Could you check a few things on this model? Use its own coordinates, in mm. A direction names the side the tool comes from. Coordinates: 2 decimals unless noted, no trailing zeros. Write each loop counter-clockwise with the first axis right and the second up, starting at its lowest first coordinate (ties: lowest second). Pieces come first, ordered by that corner, then holes. Notation, with made-up numbers: M 38,-9 L 82,-9 A20 ccw 82,18 Z; hole C 38,72 d2. An arc over 180 degrees is marked long. Answer as CSV lines item,"result". Start each with the question number.
Item 1: We'd pull the mould along X, two halves only. Please class faces 6 (the cylindrical face through (13.117, 2.07, 26.74)), 7 (the flat face through (-18.121, -3, 13)), 8 (the flat face through (-18.283, 2.3, 12.8)): +X half, -X half, draft (parallel to the pull), parting line (faces both ways), or undercut.
Item 2: On a 3-axis mill with a long thin cutter (end or side, diameter ignored), from which of +Z, -Z, +X, -X, +Y, -Y can I reach the whole of each face in a straight line? I mean faces 1 (the flat face through (-21, 1.131, 13)), 2 (the cylindrical face through (-13, -3, 3)), 3 (the flat face through (9.917, 0, 13)), 4 (the flat face through (-4, 1.907, 13)), 5 (the flat face through (-20, 2.733, 13)). Say none if no direction works.
Item 3: Suppose I cut it at C-C, the plane x = 4.5. Write out the boundary of the cut face in (y, z), and give its area (3 significant figures).
Item 4: Suppose I cut it at B-B, the plane y = -4. Write out the boundary of the cut face in (x, z).
Item 5: If I drill on line 1 along Z through (x, y) = (-7, 1.5); line 2 along Y through (x, z) = (-15.5, 23.75); line 3 along X through (y, z) = (0, 18.25), over which ranges is the centre line in solid material (lowest first)? Write a range as [from, to].
Item 6: Suppose I cut it at D-D, the plane x = -11. Write out the boundary of the cut face in (y, z), and give its area (3 significant figures).
Item 7: I'm going to push flat-ended pins straight in: P1, Ø3.5, axis at x = -12.5, y = 0.5, coming from the -Z side; P2, Ø3, axis at x = 8.5, z = 16, coming from the -Y side; P3, Ø2.5, axis at x = -22, z = 8.5, coming from the -Y side. Where does each tip first touch, or does it pass through?
Item 8: Suppose I cut it at A-A, the plane x = -17. Write out the boundary of the cut face in (y, z).
```python
from build123d import *

# Parameters (mm, degrees)
BOSS_EXTRUDE3_DEPTH = 26
FILLET6_START       = -1
FILLET6_DEPTH       = 28
BOSS_EXTRUDE5_DEPTH = 4
SKETCH6_R           = 0.5
BOSS_EXTRUDE6_DEPTH = 1.5
LPATTERN1_COUNT     = 2
LPATTERN1_PITCH     = 27.5


with BuildPart() as part:
    # Sketch4 → Boss-Extrude3 (new body)
    with BuildSketch(Plane.XY):
        with BuildLine():
            Line((-18.782676832, -0.738323828), (9.917323168, -0.738323828))
            Line((9.917323168, -0.738323828), (9.917323168, 0.761676172))
            Line((9.917323168, 0.761676172), (14.217323168, 0.761676172))
            Line((14.217323168, 0.761676172), (14.217323168, 3.761676172))
            Line((14.217323168, 3.761676172), (10.417323168, 3.761676172))
            Line((10.417323168, 3.761676172), (10.417323168, 1.907320096))
            Line((10.417323168, 1.907320096), (-18.282676832, 1.907320096))
            Line((-18.282676832, 1.907320096), (-18.282676832, 2.732812963))
            Line((-18.282676832, 2.732812963), (-21.829938074, 2.732812963))
            ThreePointArc((-21.829938074, 2.732812963), (-22.961793852, 2.121559656), (-23.782676832, 1.131166179))
            Line((-23.782676832, 1.131166179), (-18.782676832, 1.131166179))
            Line((-18.782676832, 1.131166179), (-18.782676832, -0.738323828))
        make_face()
    extrude(amount=BOSS_EXTRUDE3_DEPTH)

    # Fillet6: read off the stored shape, not the designer's step
    # Fillet6 outline → Fillet6 (cut)
    with BuildSketch(Plane.XY.offset(FILLET6_START)):
        with BuildLine():
            Line((10.417323168, 3.761676172), (10.417323168, 1.907320096))
            add(Edge.make_bspline(
                [(10.417323168, 1.907320096), (10.684335221, 2.237350554), (10.951347275, 2.567381012), (11.617088855, 3.247333717), (12.422778443, 3.640500924), (13.36841604, 3.74688263), (13.792869604, 3.754279401), (14.217323168, 3.761676172)],
                knots=[0, 0, 0, 0, 0, 0, 0.5, 0.5, 1, 1, 1, 1, 1, 1], degree=5))
            Line((14.217323168, 3.761676172), (10.417323168, 3.761676172))
        make_face()
    extrude(amount=FILLET6_DEPTH, mode=Mode.SUBTRACT)

    # Sketch5 → Boss-Extrude5 (add)
    with BuildSketch(Plane(origin=(0, -0.738323828, 0), x_dir=(-1, 0, 0), z_dir=(0, -1, 0))):
        with BuildLine():
            Line((18.120676832, -8), (18.120676832, -18))
            ThreePointArc((18.120676832, -18), (13.120676832, -23), (8.120676832, -18))
            Line((8.120676832, -18), (8.120676832, -8))
            ThreePointArc((8.120676832, -8), (13.120676832, -3), (18.120676832, -8))
        make_face()
    extrude(amount=BOSS_EXTRUDE5_DEPTH)

    # Sketch6 → Boss-Extrude6 (add)
    with BuildSketch(Plane.XY.offset(26)):
        with Locations(Location((12.617323168, 2.091676172, 0), (0, 0, 180))):
            Circle(SKETCH6_R)
    boss_extrude6 = extrude(amount=BOSS_EXTRUDE6_DEPTH)

    # LPattern1: Boss-Extrude6 ×2
    with Locations(*[(0, 0, -i * LPATTERN1_PITCH) for i in range(1, LPATTERN1_COUNT)]):
        add(boss_extrude6)


solid = part.part
```
Ans:
1,face 6,"parting line"
1,face 7,"-X half"
1,face 8,"undercut"
2,face 1,"+Z, -Z, -X, -Y"
2,face 2,"-Z, -Y"
2,face 3,"+Z, -Z, +X, -Y"
2,face 4,"+Z, -Z, +Y"
2,face 5,"+Z, -Z, -X, +Y"
3,outline,"M -0.74,0 L 1.91,0 L 1.91,26 L -0.74,26 Z"
3,area,"68.8 mm^2"
4,outline,"M -18.12,8 A5 ccw -8.12,8 L -8.12,18 A5 ccw -18.12,18 Z"
5,line 1,"z = [0, 26]"
5,line 2,"y = [-0.74, 1.91]"
5,line 3,"x = [-18.78, 9.92]"
6,outline,"M -4.74,3.47 L -0.74,3.47 L -0.74,0 L 1.91,0 L 1.91,26 L -0.74,26 L -0.74,22.53 L -4.74,22.53 Z"
6,area,"145 mm^2"
7,P1,"stops at z = 0"
7,P2,"stops at y = -0.74"
7,P3,"stops at y = 1.13"
8,outline,"M -4.74,4.85 L -0.74,4.85 L -0.74,0 L 1.91,0 L 1.91,26 L -0.74,26 L -0.74,21.15 L -4.74,21.15 Z"
